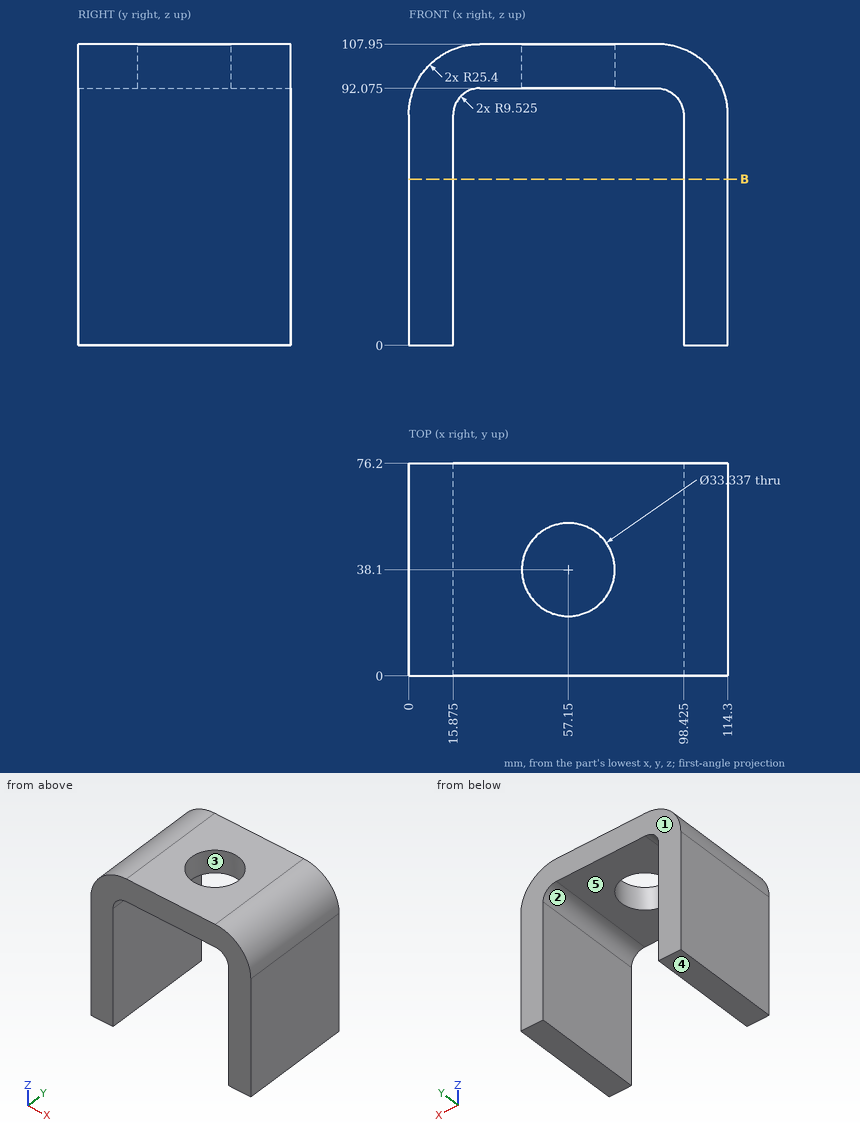
Here's the drawing with two shaded views (mm, measured from the low corner). I have some questions. A direction names the side the tool comes from. Round coordinates to 2 decimals unless told otherwise and drop trailing zeros. Order: outer loops, then holes, each group sorted by start corner. A loop starts at its lowest first (then second) coordinate and runs counter-clockwise, first axis right, second up. Notation, with made-up numbers: (83.5, -3.5) -> (113.5, -3.5) arc R21 cw to (113.5, 31.5) -> close; hole circle Ø6 at (62, 48.25). An arc over 180 degrees is marked (long way). Use a Markdown table: item, result. Add a question column.
(1) For the marked faces 4 and 5, which set-ups out of +Z, -Z, +X, -X, +Y, -Y let a thin tool reach every point of the face, with its end or its side?
(2) If we mould it in two halves opening along Y, with no side actions, what happens to the marked faces 1, 2 and 3? For each: released by +Y, released by -Y, zero draft, split by the parting line, or undercut.
(3) For pin 1 Ø5 at (y, z) = (56.5, 94.5) entering from -X; pin 2 Ø8 at (x, z) = (20.5, 57) entering from -Y (3 decimals); pin 3 Ø2 at (y, z) = (34, 90.5) entering from -X, each with a flat end and sliding along its axis, tell me the tip position at first contact or that it passes through.
(4) Suppose I cut it at B-B, the plane z = 59.5. Please give me the cut outline in (x, y) (1 decimal), and give its area (3 significant figures).
(5) I need wall thicknesses on line 1 along Y through (x, z) = (57, 97); line 2 along X through (y, z) = (24, 51) (1 decimal); line 3 along Z through (x, y) = (89.5, 43.5) (1 decimal). Which ranges of each line are inside material? Lowest first, please.
Verdict:
| question | item | result |
|---|---|---|
| 1 | face 4 | -Z, +X, -X, +Y, -Y |
| 1 | face 5 | -Z, +Y, -Y |
| 2 | face 1 | released by +Y |
| 2 | face 2 | zero draft |
| 2 | face 3 | undercut |
| 3 | pin 1 | x = 1.82 |
| 3 | pin 2 | through |
| 3 | pin 3 | x = 0.97 |
| 4 | outline | (0, 0) -> (15.9, 0) -> (15.9, 76.2) -> (0, 76.2) -> close; (98.4, 0) -> (114.3, 0) -> (114.3, 76.2) -> (98.4, 76.2) -> close |
| 4 | area | 2,420 mm2 |
| 5 | line 1 | 0 to 21.43, 54.77 to 76.2 |
| 5 | line 2 | 0 to 15.9, 98.4 to 114.3 |
| 5 | line 3 | 92.1 to 107.9 |
